Source: CAD feature listing. Evaluate the final solid. Frame: model axes, mm. A direction names the side the tool comes from. Round coordinates to 2 decimals unless told otherwise and drop trailing zeros. Loops run counter-clockwise (first coordinate to the right, second up) from the corner with the lowest first, then second, coordinate; pieces in that order, holes last. Notation, with made-up numbers: (26.25, -39.5) -> (75.25, -39.5) arc R37 cw to (75.25, -3.5) -> close; hole circle Ø11 at (9, -24). An arc over 180 degrees is marked (long way). Put each result on its own line as item: value. Start each with the question number.
1. Cut plane A-A (x = -12.5). Return the cut outline in (y, z).
2. Set-up query: faces 1 (the flat face through (0, 0, 1.6)), 2 (the flat face through (14, -8, 0)), 3 (the flat face through (-15, -8, 0)). Return all of +Z, -Z, +X, -X, +Y, -Y with unobstructed straight access to the full face (end or side cutting, diameter ignored); none if empty.
3. Contact query for flat-ended pins moving along their axis: pin 1 (1 mm diameter, centred on x = 14.5, y = -7.5, fed in from -Z); pin 2 (0.9 mm diameter, centred on y = -8, z = -0.5, fed in from -X). Output: stop coordinate, or through.
4. Material intervals for L1, parallel to X at y = 5, z = -0.3; L2, parallel to Y at x = -9.5, z = -0.55; L3, parallel to Z at x = -5, y = 8.25, sorted ascending.
5. Cut plane B-B (x = 2.5). Return the cut outline in (y, z).
```python
from build123d import *

# Parameters (mm, degrees)
SKETCH_1_W      = 31
SKETCH_1_H      = 17.6
EXTRUDE_1_DEPTH = 1.6
EXTRUDE_2_DEPTH = 0.8


with BuildPart() as part:
    # 草图1 → 凸台-拉伸1 (new body)
    with BuildSketch(Plane.XY):
        Rectangle(SKETCH_1_W, SKETCH_1_H)
    extrude(amount=EXTRUDE_1_DEPTH)

    # 草图2 → 凸台-拉伸2 (add)
    with BuildSketch(Plane(origin=(0, 0, 0), x_dir=(-1, 0, 0), z_dir=(0, 0, -1))):
        Polygon((-13.5, -8.8), (-13.5, -6.8), (-15.5, -6.8), (-15.5, 6.8), (-1, 6.8), (-1, 4.8), (3, 4.8), (3, 6.735183862), (15.5, 6.735183862), (15.5, -6.8), (13.5, -6.8), (13.5, -8.8), align=None)
    extrude(amount=EXTRUDE_2_DEPTH)


solid = part.part
```
Solution:
1. outline: (-8.8, -0.8) -> (6.74, -0.8) -> (6.74, 0) -> (8.8, 0) -> (8.8, 1.6) -> (-8.8, 1.6) -> close
2. face 1: +Z, +X, -X, +Y, -Y
2. face 2: -Z, +X, -Y
2. face 3: -Z, -X, -Y
3. pin 1: stops at z = 0
3. pin 2: stops at x = -13.5
4. L1: x = -15.5 to -3, 1 to 15.5
4. L2: y = -8.8 to 6.74
4. L3: z = 0 to 1.6
5. outline: (-8.8, -0.8) -> (6.8, -0.8) -> (6.8, 0) -> (8.8, 0) -> (8.8, 1.6) -> (-8.8, 1.6) -> close
